from build123d import *

# Parameters (mm, degrees)
SKETCH3_R           = 7.5
BOSS_EXTRUDE1_DEPTH = 3.5
SKETCH4_R           = 4
BOSS_EXTRUDE2_DEPTH = 15
BOSS_EXTRUDE4_START = 3.5
SKETCH6_R           = 4
BOSS_EXTRUDE4_DEPTH = 3.5
SKETCH7_OUTSIDE_W   = 23.112
SKETCH7_OUTSIDE_H   = 23.112
CUT_EXTRUDE1_DEPTH  = 6


with BuildPart() as part:
    # Sketch3 → Boss-Extrude1 (new body)
    with BuildSketch(Plane(origin=(0, 0, 0), x_dir=(1, 0, 0), z_dir=(0, 1, 0))):
        with Locations(Location((1.2, 0, 0), (0, 0, 270))):
            Circle(SKETCH3_R)
    extrude(amount=BOSS_EXTRUDE1_DEPTH)

    # Sketch4 → Boss-Extrude2 (add)
    with BuildSketch(Plane.XZ):
        with Locations(Location((0, 0, 0), (0, 0, 270))):
            Circle(SKETCH4_R)
    extrude(amount=BOSS_EXTRUDE2_DEPTH)

    # Sketch6 → Boss-Extrude4 (add)
    with BuildSketch(Plane(origin=(0, 3.5, 0), x_dir=(1, 0, 0), z_dir=(0, 1, 0)).offset(BOSS_EXTRUDE4_START)):
        with Locations(Location((0, 0, 0), (0, 0, 90))):
            Circle(SKETCH6_R)
    extrude(amount=-BOSS_EXTRUDE4_DEPTH)

    # Sketch7 outside → Cut-Extrude1 (cut)
    with BuildSketch(Plane.XZ.offset(15)):
        with Locations((1.2, 0)):
            Rectangle(SKETCH7_OUTSIDE_W, SKETCH7_OUTSIDE_H)
        Polygon((0, 3.666174209), (-3.175, 1.833087105), (-3.175, -1.833087105), (0, -3.666174209), (3.175, -1.833087105), (3.175, 1.833087105), align=None, mode=Mode.SUBTRACT)
    extrude(amount=-CUT_EXTRUDE1_DEPTH, mode=Mode.SUBTRACT)


solid = part.part
Part model, mm, in its own coordinate system. A direction names the side the tool comes from. Coordinates: 2 decimals unless noted, no trailing zeros. Order: outer loops, then holes, each group sorted by start corner. A loop starts at its lowest first (then second) coordinate and runs counter-clockwise, first axis right, second up.
(1) Probe L1, parallel to Y at x = -0.25, z = -6; L2, parallel to X at y = -11.25, z = -0.25 (3 decimals); L3, parallel to X at y = 1.5, z = 0.25. List the from-to ranges inside material, lowest first.
Check sheet entries:
L1: y = 0 to 3.5
L2: x = -3.175 to 3.175
L3: x = -6.3 to 8.7
(2) Slice it at B-B, the plane y = -10.75. Write the cut outline in (x, z) (3 decimals), and give its area (3 significant figures).
Check sheet entries:
outline: (-3.175, -1.833) - (0, -3.666) - (3.175, -1.833) - (3.175, 1.833) - (0, 3.666) - (-3.175, 1.833) - close
area: 34.9 mm2
(3) Pin check, flat tips, straight feed: pin 1 Ø6 at (x, y) = (-3, -10) entering from +Z; pin 2 Ø8 at (y, z) = (-1, -3.5) entering from +X; pin 3 Ø4 at (y, z) = (-12.5, -0.5) entering from -X (3 decimals); pin 4 Ø3 at (x, y) = (-3.5, -5.5) entering from +Z. Stop position of each tip, or through.
Check sheet entries:
pin 1: stops at z = 4
pin 2: stops at x = 8.7
pin 3: stops at x = -3.175
pin 4: stops at z = 3.46
(4) Tool access for faces 1 (the face through (1.57, -12.04, -2.76)), 2 (the face through (5, 0, 0)), 3 (the face through (3.905, 5.274, 0.867)), 4 (the face through (3.175, -12, 0)): list every direction of +Z, -Z, +X, -X, +Y, -Y with a clear straight run to the whole face (end or side of a thin tool).
Check sheet entries:
face 1: -Z, +X, -Y
face 2: -Y
face 3: +Y
face 4: +Z, -Z, +X, -Y
(5) Slice it at A-A, the plane z = 0. Write the cut outline in (x, y) (3 decimals).
Check sheet entries:
outline: (-6.3, 0) - (-4, 0) - (-4, -9) - (-3.175, -9) - (-3.175, -15) - (3.175, -15) - (3.175, -9) - (4, -9) - (4, 0) - (8.7, 0) - (8.7, 3.5) - (4, 3.5) - (4, 7) - (-4, 7) - (-4, 3.5) - (-6.3, 3.5) - close
(6) Slice it at C-C, the plane x = -1.5. Write the cut outline in (y, z), and give its area (3 significant figures).
Check sheet entries:
outline: (-15, -2.8) - (-9, -2.8) - (-9, -3.71) - (0, -3.71) - (0, -7) - (3.5, -7) - (3.5, -3.71) - (7, -3.71) - (7, 3.71) - (3.5, 3.71) - (3.5, 7) - (0, 7) - (0, 3.71) - (-9, 3.71) - (-9, 2.8) - (-15, 2.8) - close
area: 175 mm2
(7) Slice it at D-D, the plane y = 2.5. Write the cut outline in (x, z), and give its area (3 significant figures).
Check sheet entries:
outline: circle Ø15 at (1.2, 0)
area: 177 mm2
